from build123d import *

# Parameters (mm, degrees)
SKETCH1_W           = 60
SKETCH1_H           = 15
BOSS_EXTRUDE2_DEPTH = 20
SKETCH4_R           = 2.509766753
BOSS_EXTRUDE3_DEPTH = 20
SKETCH5_W           = 16
SKETCH5_H           = 11
BOSS_EXTRUDE4_DEPTH = 15
FILLET2_R           = 4
FILLET3_R           = 4
FILLET6_R           = 4
FILLET7_R           = 3
FILLET8_R           = 3


with BuildPart() as part:
    # Sketch1 → Boss-Extrude2 (new body)
    with BuildSketch(Plane.XY):
        with Locations((-19.125, -0.469901236)):
            Rectangle(SKETCH1_W, SKETCH1_H)
    extrude(amount=BOSS_EXTRUDE2_DEPTH)

    # Sketch4 → Boss-Extrude3 (add)
    with BuildSketch(Plane(origin=(0, 7.030098764, 0), x_dir=(1, 0, 0), z_dir=(0, 1, 0))):
        with Locations((-37.125, -10)):
            Circle(SKETCH4_R)
    extrude(amount=BOSS_EXTRUDE3_DEPTH)

    # Sketch5 → Boss-Extrude4 (add)
    with BuildSketch(Plane(origin=(10.875, 0, 0), x_dir=(0, 0, -1), z_dir=(1, 0, 0))):
        with Locations((-10, -0.469901236)):
            Rectangle(SKETCH5_W, SKETCH5_H)
    extrude(amount=BOSS_EXTRUDE4_DEPTH)

    # Fillet2
    fillet2_edges = [part.edges().sort_by_distance(p)[0] for p in [
        (18.375, 5.030098764, 2),
    ]]
    fillet(fillet2_edges, radius=FILLET2_R)

    # Fillet3
    fillet3_edges = [part.edges().sort_by_distance(p)[0] for p in [
        (18.375, 5.030098764, 18),
    ]]
    fillet(fillet3_edges, radius=FILLET3_R)

    # Fillet6
    fillet6_edges = [part.edges().sort_by_distance(p)[0] for p in [
        (18.375, -5.969901236, 2),
        (18.375, -5.969901236, 18),
    ]]
    fillet(fillet6_edges, radius=FILLET6_R)

    # Fillet7
    fillet7_edges = [part.edges().sort_by_distance(p)[0] for p in [
        (25.875, 5.030098764, 10),
        (25.875, 3.858525889, 3.171572875),
        (25.875, -0.469901236, 18),
        (25.875, 3.858525889, 16.828427125),
        (25.875, -5.969901236, 10),
        (25.875, -0.469901236, 2),
        (25.875, -4.798328361, 3.171572875),
        (25.875, -4.798328361, 16.828427125),
    ]]
    fillet(fillet7_edges, radius=FILLET7_R)

    # Fillet8
    fillet8_edges = [part.edges().sort_by_distance(p)[0] for p in [
        (-49.125, -0.469901236, 20),
        (-49.125, -0.469901236, 0),
    ]]
    fillet(fillet8_edges, radius=FILLET8_R)


solid = part.part
Geometry check sheet. Reference: the model listing, model coordinates, mm. A direction names the side the tool comes from. Give positions to 0.01 mm unless a question says otherwise; leave off trailing zeros. Write each loop counter-clockwise with the first axis right and the second up, starting at its lowest first coordinate (ties: lowest second). Pieces come first, ordered by that corner, then holes.
1) Go/stop test with flat-tipped pins: pin 1 Ø10 at (y, z) = (21, 13) entering from -X; pin 2 Ø3.5 at (x, y) = (17, -1) entering from -Z; pin 3 Ø8 at (y, z) = (16, 15) entering from -X. Record where each tip stops, or that it passes through.
Values follow:
pin 1: stops at x = -39.63
pin 2: stops at z = 2
pin 3: stops at x = -39.43
2) Set-up check for faces 1 (the face through (17, 0, 2)), 2 (the face through (17, 5.03, 10)), 3 (the face through (16.959, 3.889, 3.203)), 4 (the face through (17, -5.97, 10)): record each of +Z, -Z, +X, -X, +Y, -Y from which the full face is reachable in a straight line by a thin tool's end or side.
Values follow:
face 1: -Z, +X, +Y, -Y
face 2: +Z, -Z, +X, +Y
face 3: -Z, +X, +Y
face 4: +Z, -Z, +X, -Y
3) Cross-section at C-C (y = 18). Record the boundary of the cut face in (x, z) (3 decimals), plus the area to 3 significant figures.
Values follow:
outline: circle Ø5.02 at (-37.125, 10)
area: 19.8 mm2
4) Cross-section at B-B (x = 0). Record the boundary of the cut face in (y, z).
Values follow:
outline: (-7.97, 0) - (7.03, 0) - (7.03, 20) - (-7.97, 20) - close
5) Cross-section at A-A (z = 10). Record the boundary of the cut face in (x, y) (3 decimals).
Values follow:
outline: (-49.125, -7.97) - (10.875, -7.97) - (10.875, -5.97) - (22.875, -5.97) arc R3 ccw to (25.875, -2.97) - (25.875, 2.03) arc R3 ccw to (22.875, 5.03) - (10.875, 5.03) - (10.875, 7.03) - (-34.615, 7.03) - (-34.615, 27.03) - (-39.635, 27.03) - (-39.635, 7.03) - (-49.125, 7.03) - close
6) Thickness scan on line 1 (Y direction, x = -37.5, z = 2.5); line 2 (X direction, y = -4.5, z = 9.5) (3 decimals); line 3 (Y direction, x = 11, z = 4). Record the ranges inside material, lowest first.
Values follow:
line 1: y = -7.97 to 7.03
line 2: x = -49.125 to 25.455
line 3: y = -5.43 to 4.49
